The listing builds one solid part. Answer for the finished solid, in the listing's coordinates (mm). A direction names the side the tool comes from. Round coordinates to 2 decimals unless told otherwise and drop trailing zeros. Write each loop counter-clockwise with the first axis right and the second up, starting at its lowest first coordinate (ties: lowest second). Pieces come first, ordered by that corner, then holes. Notation, with made-up numbers: (72, 42.5) - (109, 42.5) arc R21 ccw to (109, 48.5) - close; hole circle Ø2 at (27.25, -3.75). An arc over 180 degrees is marked (long way). Return JSON: item names as keys, results as strings. Group by question number.
(1) Section A-A, the plane y = -82 is taken. Write down the section's boundary in (x, z).
(2) Section C-C, the plane y = -64.5 is taken. Write down the section's boundary in (x, z).
(3) Which of the six approach directions +Z, -Z, +X, -X, +Y, -Y give full straight-line access (tool end or side, diameter ignored) to faces 1 (the flat face through (0, -68.146, 30)), 2 (the flat face through (-38.5, -66.68, 70.14)), 3 (the cylindrical face through (0.61, -36.77, 39.44))?
(4) Find the intervals of material crossed by line 1 along Z through (x, y) = (-4, -55.5); line 2 along X through (y, z) = (-71.5, 43); line 3 along X through (y, z) = (-44.5, 61), in increasing order. Write a range as [from, to].
(5) Section B-B, the plane z = 58 is taken. Write down the section's boundary in (x, y).
(6) Determine the mould class of faces 4 (the flat face through (-1, -61, 0)), 5 (the flat face through (42.105, -64.927, 39.44)), 6 (the flat face through (-21.32, -76.93, 29.58)) for opening direction X: +X half, -X half, draft (parallel to the pull), parting line (faces both ways), or undercut.
(7) Section D-D, the plane x = 17.5 is taken. Write down the section's boundary in (y, z).
(8) Each of these flat-tipped pins is pushed along its axis until it touches: pin 1 (12 mm diameter, centred on x = -26.5, z = 18.5, fed in from +Y); pin 2 (10 mm diameter, centred on y = -59.5, z = 20.5, fed in from -X); pin 3 (2 mm diameter, centred on x = 3, z = 64, fed in from +Y). Where does it stop, or does it pass through?
```python
from build123d import *

# Parameters (mm, degrees)
F2_DEPTH = 80
F4_DEPTH = 20


with BuildPart() as f2:
    # F1 (on Top) → F2 (new body)
    with BuildSketch(Plane.XY):
        Polygon((-47.03461, -73.466334), (-26.25, -85.466334), (-16.25, -68.145826), (-37.03461, -56.145826), align=None)
        with BuildLine():
            Line((-37.03461, -56.145826), (-16.25, -68.145826))
            Line((-16.25, -68.145826), (16.25, -68.145826))
            Line((16.25, -68.145826), (37.03461, -56.145826))
            ThreePointArc((37.03461, -56.145826), (0, -36.763884), (-37.03461, -56.145826))
        make_face()
        Polygon((37.03461, -56.145826), (16.25, -68.145826), (26.25, -85.466334), (47.03461, -73.466334), align=None)
    extrude(amount=F2_DEPTH)

    # F3 (on face) → F4 (cut)
    with BuildSketch(Plane.XY.offset(80)):
        with BuildLine():
            Line((-43.570508, -75.466334), (-26.25, -85.466334))
            Line((-26.25, -85.466334), (-16.25, -68.145826))
            Line((-16.25, -68.145826), (16.25, -68.145826))
            Line((16.25, -68.145826), (26.25, -85.466334))
            Line((26.25, -85.466334), (43.570508, -75.466334))
            Line((43.570508, -75.466334), (33.570508, -58.145826))
            ThreePointArc((33.570508, -58.145826), (0, -40.748813), (-33.570508, -58.145826))
            Line((-33.570508, -58.145826), (-43.570508, -75.466334))
        make_face()
    extrude(amount=-F4_DEPTH, mode=Mode.SUBTRACT)


solid = f2.part
```
Working result:
{
 "1": {"outline": "(-32.25, 0) - (-24.25, 0) - (-24.25, 60) - (-32.25, 60) - close; (24.25, 0) - (32.25, 0) - (32.25, 60) - (24.25, 60) - close"},
 "2": {"outline": "(-41.86, 0) - (41.86, 0) - (41.86, 80) - (37.24, 80) - (37.24, 60) - (-37.24, 60) - (-37.24, 80) - (-41.86, 80) - close"},
 "3": {"face 1": "+Z, -Z, -Y", "face 2": "+Z, -Y", "face 3": "+Z, -Z, +Y"},
 "4": {"line 1": "z = [0, 60]", "line 2": "x = [-45.9, -18.19], [18.19, 45.9]", "line 3": "x = [-25.25, -17.15], [17.15, 25.25]"},
 "5": {"outline": "(-47.03, -73.47) - (-26.25, -85.47) - (-16.25, -68.15) - (16.25, -68.15) - (26.25, -85.47) - (47.03, -73.47) - (37.03, -56.15) arc R45.07 ccw to (-37.03, -56.15) - close"},
 "6": {"face 4": "draft", "face 5": "+X half", "face 6": "undercut"},
 "7": {"outline": "(-70.31, 0) - (-40.3, 0) - (-40.3, 80) - (-44.66, 80) - (-44.66, 60) - (-70.31, 60) - close"},
 "8": {"pin 1": "stops at y = -41.7", "pin 2": "stops at x = -41.86", "pin 3": "stops at y = -36.81"}
}
